For this review, use the dimensioned drawing (mm, ordinates from the lowest corner) and the shaded views. Give positions to 0.01 mm unless a question says otherwise; leave off trailing zeros. Write each loop counter-clockwise with the first axis right and the second up, starting at its lowest first coordinate (ties: lowest second). Pieces come first, ordered by that corner, then holes. Notation, with made-up numbers: (63, -7.5) -> (81, -7.5) arc R21 ccw to (81, 28.5) -> close; hole circle Ø1 at (14, 47.5). An arc over 180 degrees is marked (long way). Answer as CSV lines item,"result".
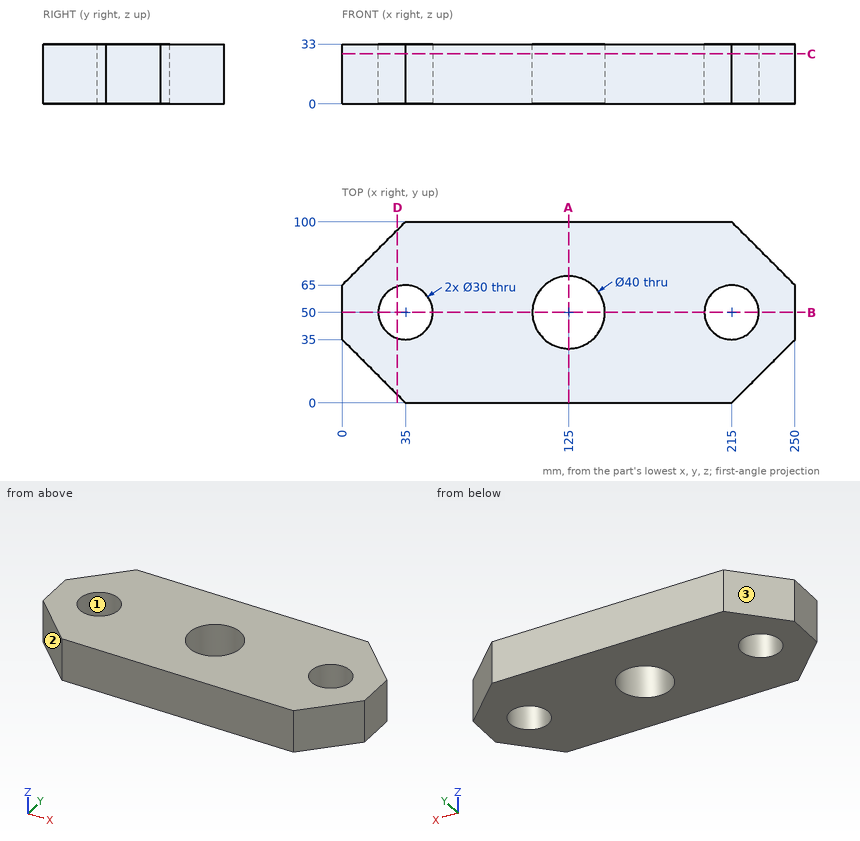
Q1. Add section D-D (x = 30.5). Write out the cut boundary in (y, z).
Answer block:
outline,"(4.5, 0) -> (35.69, 0) -> (35.69, 33) -> (4.5, 33) -> close; (64.31, 0) -> (95.5, 0) -> (95.5, 33) -> (64.31, 33) -> close"
Q2. To check wall thickness, follow probe 1 along Y at (x, z) = (117.5, 8); probe 2 along X at (y, z) = (40.5, 4.5); probe 3 along X at (y, z) = (66, 22.5). State the ranges of each line that lie inside material, in increasing order. Write a range as [from, to].
Answer block:
probe 1,"y = [0, 31.46], [68.54, 100]"
probe 2,"x = [0, 23.39], [46.61, 107.4], [142.6, 203.39], [226.61, 250]"
probe 3,"x = [1, 113], [137, 249]"
Q3. Add section B-B (y = 50). Write out the cut boundary in (x, z), plus the area to 3 significant figures.
Answer block:
outline,"(0, 0) -> (20, 0) -> (20, 33) -> (0, 33) -> close; (50, 0) -> (105, 0) -> (105, 33) -> (50, 33) -> close; (145, 0) -> (200, 0) -> (200, 33) -> (145, 33) -> close; (230, 0) -> (250, 0) -> (250, 33) -> (230, 33) -> close"
area,"4,950 mm2"
Q4. Draft analysis for pull direction Y (two halves, no side actions). For the marked faces 1, 2 and 3, state which applies: released by +Y, released by -Y, zero draft, split by the parting line, or undercut.
Answer block:
face 1,"undercut"
face 2,"released by -Y"
face 3,"released by +Y"
Q5. Clearance check with a flat-ended pin moving along its axis: pin 1 (1.5 mm diameter, centred on y = 82.5, z = 28, fed in from +X). State where the tip first meets the part, or that it passes through.
Answer block:
pin 1,"stops at x = 233.25"
Q6. Add section C-C (z = 27.5). Write out the cut boundary in (x, y).
Answer block:
outline,"(0, 35) -> (35, 0) -> (215, 0) -> (250, 35) -> (250, 65) -> (215, 100) -> (35, 100) -> (0, 65) -> close; hole circle Ø30 at (35, 50); hole circle Ø40 at (125, 50); hole circle Ø30 at (215, 50)"
Q7. Add section A-A (x = 125). Write out the cut boundary in (y, z), plus the area to 3 significant figures.
Answer block:
outline,"(0, 0) -> (30, 0) -> (30, 33) -> (0, 33) -> close; (70, 0) -> (100, 0) -> (100, 33) -> (70, 33) -> close"
area,"1,980 mm2"
